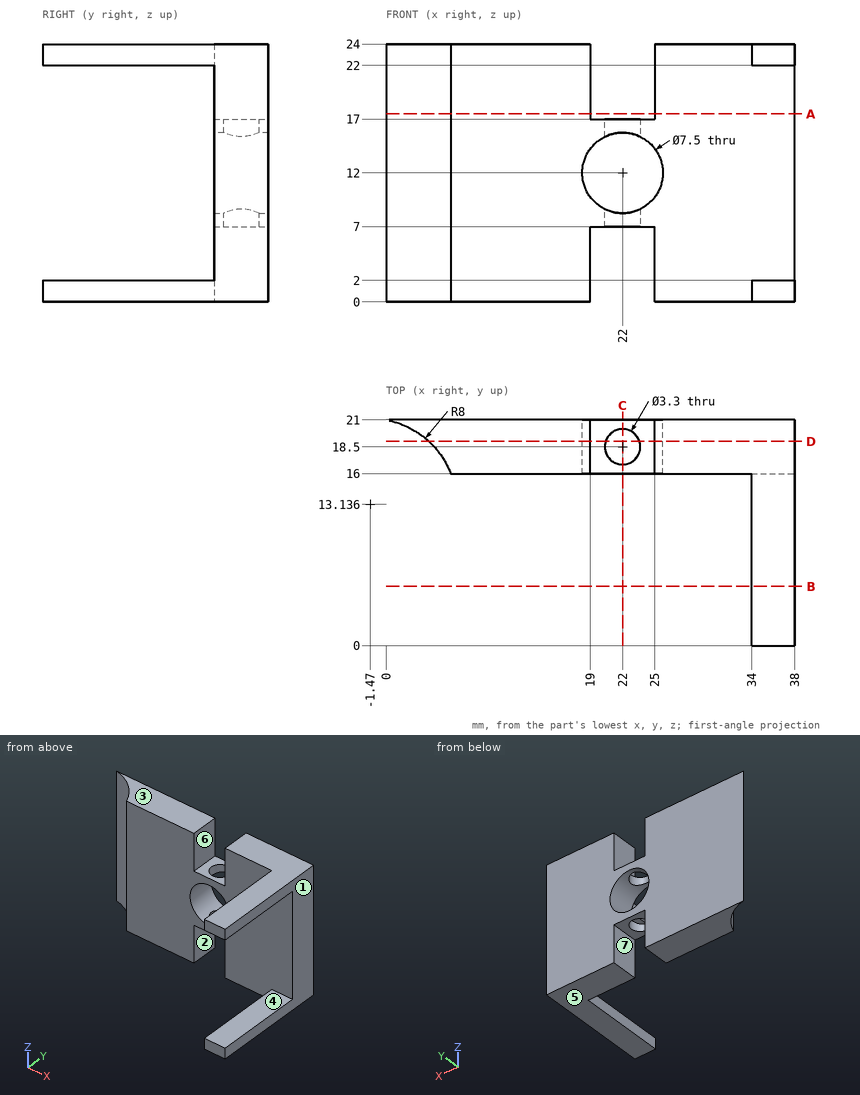
Geometry check sheet. Reference: drawing and pictorial views, mm from the part's lowest x, y, z. A direction names the side the tool comes from. Round coordinates to 2 decimals unless told otherwise and drop trailing zeros. Loops run counter-clockwise (first coordinate to the right, second up) from the corner with the lowest first, then second, coordinate; pieces in that order, holes last. Notation, with made-up numbers: (11, 6.25) - (36, 6.25) arc R32 ccw to (36, 36.25) - close; hole circle Ø1 at (85, 21). An arc over 180 degrees is marked (long way). Write item = value, one per line. Start each with the question number.
Q1. Depth check by flat-ended pin: P1, Ø5, axis at y = 17, z = 14, coming from the -X side; P2, Ø12, axis at x = 12, z = 20, coming from the -Y side; P3, Ø2.5, axis at y = 17.5, z = 3.5, coming from the -X side. Enter the tip coordinate at first touch or a pass-through.
Q2. Release check for a two-part mould opening along X. For the marked faces 1, 2 and 3 record: pulls with the +X half, pulls with the -X half, needs draft (parallel to the pull), parting line crosses it, or undercut.
Q3. Access from +Z, -Z, +X, -X, +Y, -Y to the whole of each face (thin tool, end or side, straight path). Record for the marked faces 4, 5, 6 and 7.
Q4. Thickness scan on L1, parallel to Y at x = 22, z = 15.9; L2, parallel to Y at x = 2, z = 21.5 (1 decimal); L3, parallel to Y at x = 8, z = 14.25. Record the ranges inside material, lowest first.
Q5. Section check C-C (x = 22). Record the boundary of the cut face in (y, z).
Q6. Section check D-D (y = 19). Record the boundary of the cut face in (x, z), plus the area to 3 significant figures.
Q7. Section check A-A (z = 17.5). Record the boundary of the cut face in (x, y), plus the area to 3 significant figures.
Q8. Section check B-B (y = 5.5). Record the boundary of the cut face in (x, z).
Derived:
q1.P1 = 3.38
q1.P2 = 16
q1.P3 = 4.23
q2.face_1 = pulls with the +X half
q2.face_2 = undercut
q2.face_3 = needs draft
q3.face_4 = +X, -X, -Y
q3.face_5 = -Z, +X, -X, +Y, -Y
q3.face_6 = +Z, +Y, -Y
q3.face_7 = -Z, +Y, -Y
q4.L1 = 16 to 16.85, 20.15 to 21
q4.L2 = 20.3 to 21
q4.L3 = 16 to 21
q5.outline = (16, 7) - (16.85, 7) - (16.85, 8.25) - (16, 8.25) - close; (16, 15.75) - (16.85, 15.75) - (16.85, 17) - (16, 17) - close; (20.15, 7) - (21, 7) - (21, 8.25) - (20.15, 8.25) - close; (20.15, 15.75) - (21, 15.75) - (21, 17) - (20.15, 17) - close
q6.outline = (3.97, 0) - (19, 0) - (19, 7) - (20.43, 7) - (20.43, 8.6) arc R3.75 cw to (20.43, 15.4) - (20.43, 17) - (19, 17) - (19, 24) - (3.97, 24) - close; (23.57, 7) - (25, 7) - (25, 0) - (38, 0) - (38, 24) - (25, 24) - (25, 17) - (23.57, 17) - (23.57, 15.4) arc R3.75 cw to (23.57, 8.6) - close
q6.area = 680 mm^2
q7.outline = (0, 21) arc R8 cw to (6, 16) - (19, 16) - (19, 21) - close; (25, 16) - (38, 16) - (38, 21) - (25, 21) - close
q7.area = 140 mm^2
q8.outline = (34, 0) - (38, 0) - (38, 2) - (34, 2) - close; (34, 22) - (38, 22) - (38, 24) - (34, 24) - close
